Can you work these out from the model? Positions are in its coordinate system, mm. Face numbers are marked on the shaded views. A direction names the side the tool comes from. Give positions to 0.01 mm unless a question says otherwise; leave off trailing zeros. Write each loop counter-clockwise with the first axis right and the second up, starting at its lowest first coordinate (ties: lowest second). Pieces come first, ordered by that corner, then holes. Notation, with made-up numbers: (-29.5, -34) -> (19.5, -34) arc R10 cw to (19.5, -24) -> close; hole circle Ø9 at (-8, 61.25). An arc over 180 degrees is marked (long way). Answer as CSV lines item,"result". Start each with the question number.
1. I need wall thicknesses on line 1 (X direction, y = 26, z = 0); line 2 (Z direction, x = 0, y = 26); line 3 (Y direction, x = -11.5, z = -32.5). Which ranges of each line are inside material? Lowest first, please. Write a range as [from, to].
2. On a 3-axis mill with a long thin cutter (end or side, diameter ignored), from which of +Z, -Z, +X, -X, +Y, -Y can I reach the whole of each face in a straight line? I mean the marked faces 5, 6 and 7. Say none if no direction works.
3. If we mould it in two halves opening along Z, with no side actions, what happens to the marked faces 1, 2, 3 and 4? For each: pulls with the +Z half, pulls with the -Z half, needs draft (parallel to the pull), parting line crosses it, or undercut.
4. If we section it at A-A on y = 24: Write out the boundary of the cut face in (x, z), plus the area to 3 significant figures.
5. If we section it at D-D on x = -16: Write out the boundary of the cut face in (y, z), plus the area to 3 significant figures.
6. I'm going to push flat-ended pins straight in: P1, Ø12, axis at x = -6, y = 2.5, coming from the -Z side; P2, Ø5, axis at x = -8, y = -27, coming from the +Z side; P3, Ø13, axis at x = 0, y = 24, coming from the -Z side. Where does each tip first touch, or does it pass through?
7. If we section it at C-C on z = 4: Write out the boundary of the cut face in (x, y), plus the area to 3 significant figures.
8. If we section it at B-B on x = 0: Write out the boundary of the cut face in (y, z).
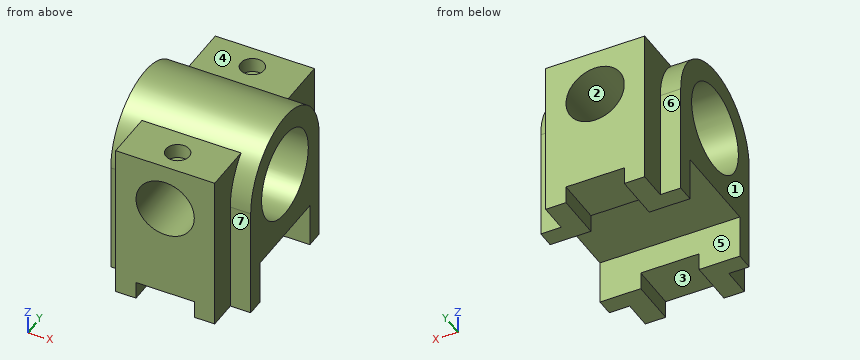
Solid Edge part; units mm, degrees
sketch "Sketch1" plane through (0, 0, 0) normal (1, 0, 0) x (0, 1, 0)
  line L0 (22, -38) -> (22, 0)
  line L1 (16, -38) -> (22, -38)
  line L2 (16, -23) -> (16, -38)
  line L3 (-16, -23) -> (16, -23)
  line L4 (-16, -38) -> (-16, -23)
  line L5 (-22, -38) -> (-16, -38)
  line L6 (-22, 0) -> (-22, -38)
  arc A0 (-22, 0) -> (22, 0) centre (0, 0) cw
  circle A1 centre (0, 0) radius 15
extrude "Protrusion1" add sketch "Sketch1" along normal mid plane 48
sketch "Sketch2" plane through (0, 0, 0) normal (0, -1, 0) x (1, 0, 0)
  line L0 (0, -32) -> (-10, -32)
  line L1 (-10, -32) -> (-10, -38)
  line L2 (-10, -38) -> (-17, -38)
  line L3 (-17, -38) -> (-17, 16)
  line L4 (-17, 16) -> (17, 16)
  line L5 (17, 16) -> (17, -38)
  line L6 (17, -38) -> (10, -38)
  line L7 (10, -38) -> (10, -32)
  line L8 (10, -32) -> (0, -32)
  circle A0 centre (0, 0) radius 10
extrude "ExtrudedProtrusion_3" add sketch "Sketch2" along normal mid plane 64
sketch "Sketch3" plane through (0, 0, 0) normal (1, 0, 0) x (0, 1, 0)
  circle A0 centre (0, 0) radius 15
extrude "ExtrudedCutout_1" cut sketch "Sketch3" along normal mid plane 64
sketch "Sketch4" plane through (0, 0, 0) normal (0, -1, 0) x (1, 0, 0)
  circle A0 centre (0, 0) radius 10
extrude "ExtrudedCutout_2" cut sketch "Sketch4" along normal mid plane 64
sketch "Sketch5" plane through (24, 0, -8) normal (1, 0, 0) x (0, 1, 0)
  line L0 (-16, -15) -> (16, -15)
  line L1 (16, -15) -> (16, -30)
  line L2 (16, -30) -> (-16, -30)
  line L3 (-16, -30) -> (-16, -15)
extrude "ExtrudedCutout_3" cut sketch "Sketch5" against normal blind 48
sketch "Sketch6" plane through (0, 32, -11) normal (0, 1, 0) x (0, 0, -1)
  line L0 (21, 10) -> (21, -10)
  line L1 (21, -10) -> (27, -10)
  line L2 (27, -10) -> (27, 10)
  line L3 (27, 10) -> (21, 10)
extrude "ExtrudedCutout_4" cut sketch "Sketch6" against normal blind 64
sketch "Sketch7" plane through (0, -23.5498, 16) normal (0, 0, 1) x (0, 1, 0)
  circle A0 centre (-0.4502, 0) radius 4
  circle A1 centre (47.5498, 0) radius 4
extrude "ExtrudedCutout_8" cut sketch "Sketch7" against normal blind 5
Computed values:
1,line 1,"x = [-17, -10], [10, 17]"
1,line 2,"z = [-32, -10], [10, 11]"
1,line 3,"y = [-32, -16], [16, 32]"
2,face 5,"-Z, +X, -X"
2,face 6,"+Z, -Z, -X, +Y"
2,face 7,"+Z, -Z, +X, -Y"
3,face 1,"needs draft"
3,face 2,"undercut"
3,face 3,"pulls with the -Z half"
3,face 4,"pulls with the +Z half"
4,outline,"(-17, -38) -> (-10, -38) -> (-10, -32) -> (10, -32) -> (10, -38) -> (17, -38) -> (17, 16) -> (4, 16) -> (4, 11) -> (-4, 11) -> (-4, 16) -> (-17, 16) -> close; hole circle Ø20 at (0, 0)"
4,area,"1,360 mm2"
5,outline,"(-32, -38) -> (-16, -38) -> (-16, -23) -> (16, -23) -> (16, -38) -> (32, -38) -> (32, 16) -> (15.1, 16) arc R22 ccw to (-15.1, 16) -> (-32, 16) -> close; hole circle Ø30 at (0, 0)"
5,area,"2,390 mm2"
6,P1,"stops at z = -23"
6,P2,"stops at z = 16"
6,P3,"stops at z = -32"
7,outline,"(-24, -21.63) -> (-17, -21.63) -> (-17, -32) -> (-9.17, -32) -> (-9.17, -14.46) -> (-24, -14.46) -> close; (-24, 14.46) -> (-9.17, 14.46) -> (-9.17, 32) -> (-17, 32) -> (-17, 21.63) -> (-24, 21.63) -> close; (9.17, -32) -> (17, -32) -> (17, -21.63) -> (24, -21.63) -> (24, -14.46) -> (9.17, -14.46) -> close; (9.17, 14.46) -> (24, 14.46) -> (24, 21.63) -> (17, 21.63) -> (17, 32) -> (9.17, 32) -> close"
7,area,"751 mm2"
8,outline,"(-32, -32) -> (-16, -32) -> (-16, -23) -> (16, -23) -> (16, -32) -> (32, -32) -> (32, -10) -> (11.18, -10) arc R15 cw to (-11.18, -10) -> (-32, -10) -> close; (-32, 10) -> (-11.18, 10) arc R15 cw to (11.18, 10) -> (32, 10) -> (32, 16) -> (28, 16) -> (28, 11) -> (20, 11) -> (20, 16) -> (15.1, 16) arc R22 ccw to (-15.1, 16) -> (-20, 16) -> (-20, 11) -> (-28, 11) -> (-28, 16) -> (-32, 16) -> close"
